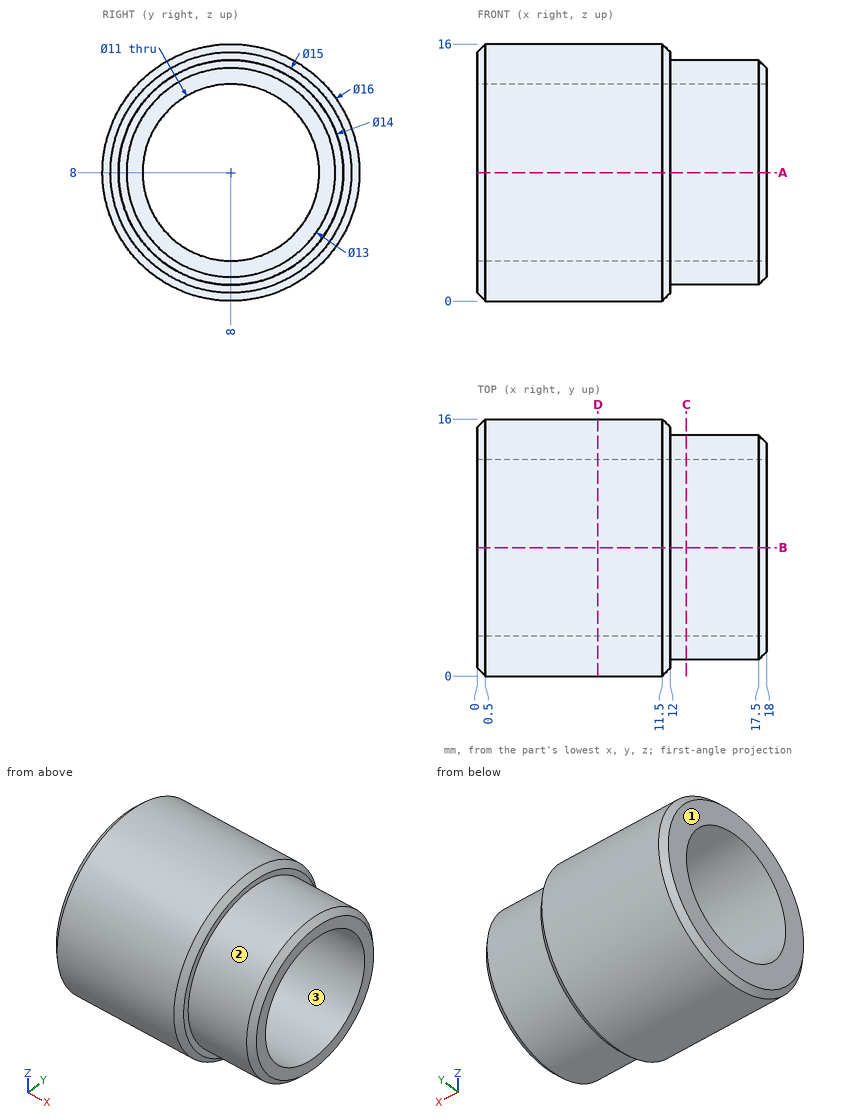
Could you check a few things on this drawing? It's one solid part, dimensions in mm from its lowest x, y, z. Give positions to 0.01 mm unless a question says otherwise; leave off trailing zeros. Write each loop counter-clockwise with the first axis right and the second up, starting at its lowest first coordinate (ties: lowest second). Pieces come first, ordered by that corner, then holes. Notation, with made-up numbers: (84, 77.5) -> (123, 77.5) arc R17 ccw to (123, 86.5) -> close; hole circle Ø11 at (79.25, -15). An arc over 180 degrees is marked (long way). Answer as CSV lines item,"result". Start each with the question number.
(1) If we section it at D-D, the plane x = 7.5: Write out the boundary of the cut face in (y, z).
(2) Please list where these lines run through material, in increasing order: line 1 (Y direction, x = 13, z = 8); line 2 (Y direction, x = 9, z = 8); line 3 (Z direction, x = 10, y = 7.5).
(3) I'm going to push flat-ended pins straight in: pin 1 Ø3 at (x, y) = (14, 3) entering from -Z; pin 2 Ø5 at (x, y) = (3, 11) entering from -Z; pin 3 Ø6 at (x, z) = (9, 8.5) entering from +Y; pin 4 Ø2 at (x, z) = (8, 12) entering from +Y. Where does each tip first touch, or does it pass through?
(4) If we mould it in two halves opening along Z, with no side actions, what happens to the marked faces 1, 2 and 3? For each: +Z half, -Z half, draft (parallel to the pull), parting line (faces both ways), or undercut.
(5) If we section it at A-A, the plane z = 8: Write out the boundary of the cut face in (x, y).
(6) If we section it at C-C, the plane x = 13: Write out the boundary of the cut face in (y, z), and give its area (3 significant figures).
Answer list:
1,outline,"circle Ø16 at (8, 8); hole circle Ø11 at (8, 8)"
2,line 1,"1 to 2.5, 13.5 to 15"
2,line 2,"0 to 2.5, 13.5 to 16"
2,line 3,"0.02 to 2.52, 13.48 to 15.98"
3,pin 1,"z = 1.94"
3,pin 2,"z = 0.02"
3,pin 3,"y = 16"
3,pin 4,"y = 15.42"
4,face 1,"draft"
4,face 2,"parting line"
4,face 3,"undercut"
5,outline,"(0, 0.5) -> (0.5, 0) -> (11.5, 0) -> (12, 0.5) -> (12, 1) -> (17.5, 1) -> (18, 1.5) -> (18, 2.5) -> (0, 2.5) -> close; (0, 13.5) -> (18, 13.5) -> (18, 14.5) -> (17.5, 15) -> (12, 15) -> (12, 15.5) -> (11.5, 16) -> (0.5, 16) -> (0, 15.5) -> close"
6,outline,"circle Ø14 at (8, 8); hole circle Ø11 at (8, 8)"
6,area,"58.9 mm^2"
